from build123d import *

# Parameters (mm, degrees)
MAIN_EXTRUSION_DEPTH    = 4
CORNER_LEAVE_R          = 5
ESQUISSE2_R             = 3
ESQUISSE2_W             = 25
ESQUISSE2_H             = 65
ENL_V_MAT_EXTRU_1_DEPTH = 267.30058205
D_GAGEMENT_M41_D        = 4.5
D_GAGEMENT_M42_D        = 4.5
D_GAGEMENT_M2_51_D      = 2.9


with BuildPart() as part:
    # Main scetch → Main extrusion (new body)
    with BuildSketch(Plane(origin=(0, 0, 0), x_dir=(1, 0, 0), z_dir=(0, 1, 0))):
        Polygon((-150, 0), (150, 0), (150, 175), (105, 220), (-105, 220), (-150, 175), align=None)
    extrude(amount=MAIN_EXTRUSION_DEPTH)

    # Corner leave
    corner_leave_edges = [part.edges().sort_by_distance(p)[0] for p in [
        (150, 2, 0),
        (-150, 2, 0),
        (-150, 2, -175),
        (-105, 2, -220),
        (105, 2, -220),
        (150, 2, -175),
    ]]
    fillet(corner_leave_edges, radius=CORNER_LEAVE_R)

    # Esquisse2 → Enlèv. mat.-Extru.1 (cut, through all)
    with BuildSketch(Plane(origin=(0, 4, 0), x_dir=(1, 0, 0), z_dir=(0, 1, 0))):
        with Locations(Location((117.47, 182.47, 0), (0, 0, 270))):
            Circle(ESQUISSE2_R)
        with Locations(Location((117.47, 137.53, 0), (0, 0, 90))):
            Circle(ESQUISSE2_R)
        with Locations(Location((-117.47, 137.53, 0), (0, 0, 270))):
            Circle(ESQUISSE2_R)
        with Locations(Location((-117.47, 182.47, 0), (0, 0, 90))):
            Circle(ESQUISSE2_R)
        with Locations((70, 160)):
            Rectangle(ESQUISSE2_W, ESQUISSE2_H)
        Polygon((100, 137.5), (100, 182.5), (111, 182.5), (111, 175), (127, 175), (127, 145), (111, 145), (111, 137.5), align=None)
        Polygon((-111, 137.5), (-111, 145), (-127, 145), (-127, 175), (-111, 175), (-111, 182.5), (-100, 182.5), (-100, 137.5), align=None)
        with Locations((-70, 160)):
            Rectangle(ESQUISSE2_W, ESQUISSE2_H)
    extrude(amount=-ENL_V_MAT_EXTRU_1_DEPTH, mode=Mode.SUBTRACT)

    # Dégagement M41 (through all)
    with Locations(Plane(origin=(0, 4, 0), x_dir=(1, 0, 0), z_dir=(0, 1, 0))):
        with Locations((-125, 30), (125, 15)):
            Hole(D_GAGEMENT_M41_D / 2)

    # Dégagement M42 (through all)
    with Locations(Plane(origin=(0, 4, 0), x_dir=(1, 0, 0), z_dir=(0, 1, 0))):
        with Locations((-142, 8), (0, 8), (142, 8), (142, 170), (-142, 170)):
            Hole(D_GAGEMENT_M42_D / 2)

    # Dégagement M2.51 (through all)
    with Locations(Plane(origin=(0, 4, 0), x_dir=(1, 0, 0), z_dir=(0, 1, 0))):
        with Locations((-125, 47.5), (-125, 12.5)):
            Hole(D_GAGEMENT_M2_51_D / 2)


solid = part.part
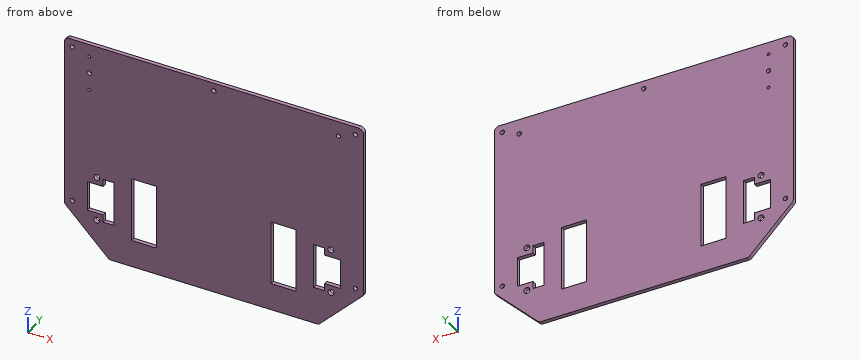
Could you check a few things on this model? Use its own coordinates, in mm. Give positions to 0.01 mm unless a question says otherwise; leave off trailing zeros. Loops run counter-clockwise (first coordinate to the right, second up) from the corner with the lowest first, then second, coordinate; pieces in that order, holes last. Notation, with made-up numbers: (49.5, 64.25) -> (84.5, 64.25) arc R31 cw to (84.5, 88.25) -> close; hole circle Ø10 at (47.25, 56). An arc over 180 degrees is marked (long way). Answer as CSV lines item,"result". Start each with the question number.
(1) I need wall thicknesses on probe 1 along X at (y, z) = (1.55, -166); probe 2 along X at (y, z) = (2.45, -47.5); probe 3 along X at (y, z) = (2.9, -184.5). Which ranges of each line are inside material? Lowest first, please.
(2) If we section it at A-A on x = -117.47: Write out the boundary of the cut face in (y, z), then the cut area to 3 significant figures.
(3) If we section it at C-C on y = 2.9: Count the separate pieces of the cut face and the enclosed holes in it, then the cut area to 3 significant figures.
(4) I'm going to push a flat-ended pin straight in: pin 1 Ø2 at (x, y) = (105.5, 2) entering from -Z. Where does the tip first touch, or does it pass through?
(5) If we section it at B-B on z = -161.5: Write out the boundary of the cut face in (x, y).
Computed:
1,probe 1,"x = -150 to -127, -100 to -82.5, -57.5 to 57.5, 82.5 to 100, 127 to 150"
1,probe 2,"x = -150 to -126.45, -123.55 to 150"
1,probe 3,"x = -140.5 to -119.68, -115.26 to -82.5, -57.5 to 57.5, 82.5 to 115.26, 119.68 to 140.5"
2,outline,"(0, -207.53) -> (4, -207.53) -> (4, -185.47) -> (0, -185.47) -> close; (0, -179.47) -> (4, -179.47) -> (4, -175) -> (0, -175) -> close; (0, -145) -> (4, -145) -> (4, -140.53) -> (0, -140.53) -> close; (0, -134.53) -> (4, -134.53) -> (4, 0) -> (0, 0) -> close"
2,area,"662 mm2"
3,separate pieces,"1"
3,enclosed holes,"17"
3,area,"58,500 mm2"
4,pin 1,"stops at z = -219.75"
5,outline,"(-150, 0) -> (-127, 0) -> (-127, 4) -> (-150, 4) -> close; (-100, 0) -> (-82.5, 0) -> (-82.5, 4) -> (-100, 4) -> close; (-57.5, 0) -> (57.5, 0) -> (57.5, 4) -> (-57.5, 4) -> close; (82.5, 0) -> (100, 0) -> (100, 4) -> (82.5, 4) -> close; (127, 0) -> (150, 0) -> (150, 4) -> (127, 4) -> close"
